Geometry: see drawing. Coordinates: mm, zero at the bounding-box minimum. A direction names the side the tool comes from. Round coordinates to 2 decimals unless told otherwise and drop trailing zeros. Loops run counter-clockwise (first coordinate to the right, second up) from the corner with the lowest first, then second, coordinate; pieces in that order, holes last.
(1) First-contact query: pin 1 Ø1.5 at (y, z) = (2, 2) entering from +X. Flat tip, straight axial feed; report the tip coordinate or a pass-through.
(2) Material intervals for probe 1 along Z at (x, y) = (3.25, 0.7); probe 2 along X at (y, z) = (1.65, 17.5); probe 3 along Z at (x, y) = (4.25, 1.05), sorted ascending.
(3) Section D-D, the plane x = 5. Return the cut outline in (y, z), plus the area to 3 significant figures.
(4) Mould query, pull axis X, two halves, no side actions, for the marked faces 1, 2, 3 and 4. Classes: pulls with the +X half, pulls with the -X half, needs draft (parallel to the pull), parting line crosses it, or undercut.
(5) Set-up query: the marked faces 5 and 6. Return all of +Z, -Z, +X, -X, +Y, -Y with unobstructed straight access to the full face (end or side cutting, diameter ignored); none if empty.
(6) Section A-A, the plane x = 3.4. Return the cut outline in (y, z).
(7) Section B-B, the plane y = 0.6. Return the cut outline in (x, z).
(8) Section C-C, the plane z = 2. Return the cut outline in (x, y), plus the area to 3 significant figures.
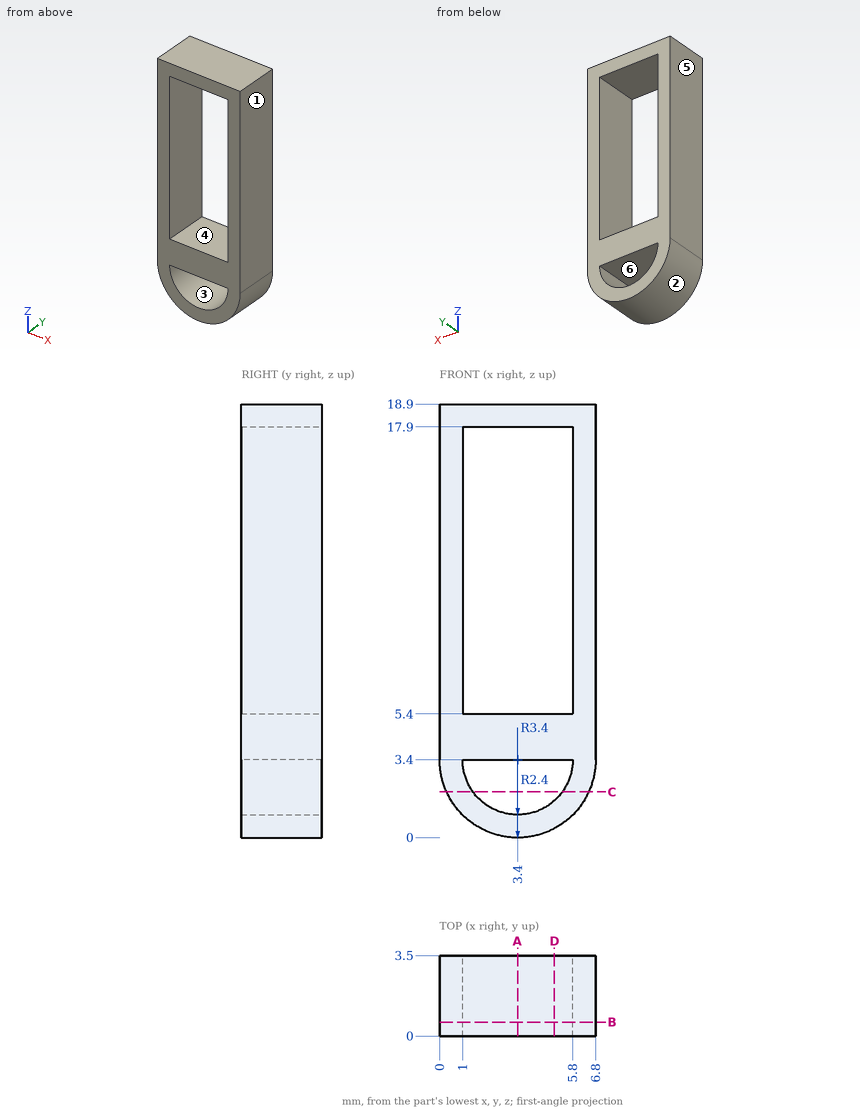
Output values:
1. pin 1: stops at x = 6.74
2. probe 1: z = 0 to 1, 3.4 to 5.4, 17.9 to 18.9
2. probe 2: x = 0 to 1, 5.8 to 6.8
2. probe 3: z = 0.11 to 1.16, 3.4 to 5.4, 17.9 to 18.9
3. outline: (0, 0.4) - (3.5, 0.4) - (3.5, 1.61) - (0, 1.61) - close; (0, 3.4) - (3.5, 3.4) - (3.5, 5.4) - (0, 5.4) - close; (0, 17.9) - (3.5, 17.9) - (3.5, 18.9) - (0, 18.9) - close
3. area: 14.7 mm2
4. face 1: pulls with the +X half
4. face 2: parting line crosses it
4. face 3: undercut
4. face 4: undercut
5. face 5: +Z, -Z, -X, +Y, -Y
5. face 6: +Y, -Y
6. outline: (0, 0) - (3.5, 0) - (3.5, 1) - (0, 1) - close; (0, 3.4) - (3.5, 3.4) - (3.5, 5.4) - (0, 5.4) - close; (0, 17.9) - (3.5, 17.9) - (3.5, 18.9) - (0, 18.9) - close
7. outline: (0, 3.4) arc R3.4 ccw to (6.8, 3.4) - (6.8, 18.9) - (0, 18.9) - close; hole (1, 3.4) arc R2.4 ccw to (5.8, 3.4) - close; hole (1, 5.4) - (5.8, 5.4) - (5.8, 17.9) - (1, 17.9) - close
8. outline: (0.3, 0) - (1.45, 0) - (1.45, 3.5) - (0.3, 3.5) - close; (5.35, 0) - (6.5, 0) - (6.5, 3.5) - (5.35, 3.5) - close
8. area: 8.04 mm2
